```python
from build123d import *

# Parameters (mm, degrees)
SKETCH1_R           = 9.525
BOSS_EXTRUDE1_DEPTH = 76.2
SKETCH3_R           = 8.509
CUT_EXTRUDE1_DEPTH  = 1.524
SKETCH4_R           = 8.001
CUT_EXTRUDE2_DEPTH  = 75.676
SKETCH5_R           = 12.4206
CUT_EXTRUDE3_DEPTH  = 254


with BuildPart() as part:
    # Sketch1 → Boss-Extrude1 (new body)
    with BuildSketch(Plane(origin=(0, 0, 0), x_dir=(0, 0, -1), z_dir=(1, 0, 0))):
        Circle(SKETCH1_R)
    extrude(amount=BOSS_EXTRUDE1_DEPTH)

    # Sketch3 → Cut-Extrude1 (cut)
    with BuildSketch(Plane.ZY):
        Circle(SKETCH3_R)
    extrude(amount=-CUT_EXTRUDE1_DEPTH, mode=Mode.SUBTRACT)

    # Sketch4 → Cut-Extrude2 (cut, through all)
    with BuildSketch(Plane.ZY.offset(-1.524)):
        Circle(SKETCH4_R)
    extrude(amount=-CUT_EXTRUDE2_DEPTH, mode=Mode.SUBTRACT)

    # Sketch5 → Cut-Extrude3 (cut)
    with BuildSketch(Plane.XY.offset(9.525)):
        with Locations((76.2, 0)):
            Circle(SKETCH5_R)
    extrude(amount=-CUT_EXTRUDE3_DEPTH, mode=Mode.SUBTRACT)


solid = part.part
```
The model under review builds one solid part; all positions refer to its coordinate system, in mm. A direction names the side the tool comes from. Coordinates: 2 decimals unless noted, no trailing zeros. Write each loop counter-clockwise with the first axis right and the second up, starting at its lowest first coordinate (ties: lowest second). Pieces come first, ordered by that corner, then holes. Notation, with made-up numbers: (22.25, 47) -> (47.25, 47) arc R19 cw to (47.25, 81) -> close; hole circle Ø5 at (82.5, 20.5). An arc over 180 degrees is marked (long way). One line per item, written item: value. Start each with the question number.
Q1. Add section A-A, the plane y = 0. Give the boundary of the cut face in (x, z) (3 decimals), then the cut area to 3 significant figures.
Q2. Clearance check with flat-ended pins moving along their axes: P1, Ø3, axis at y = 2, z = -5, coming from the +X side; P2, Ø5, axis at x = 52.5, y = 6, coming from the +Z side; P3, Ø10, axis at y = 4, z = -4, coming from the +X side; P4, Ø4, axis at x = 48, y = 6.5, coming from the -Z side (3 decimals). State where each tip first meets the part, or that it passes through.
Q3. Add section C-C, the plane x = 63. Give the boundary of the cut face in (y, z) (3 decimals).
Q4. Add section B-B, the plane z = 0. Give the boundary of the cut face in (x, y) (3 decimals).
Q5. For faces 4 (the face through (33.66, -7.81, -1.73)), 5 (the face through (0.751, 8.437, -1.108)), list the 3-axis set-ups (+Z, -Z, +X, -X, +Y, -Y) from which the entire face can be reached by the end or side of a thin tool; tool diameter is ignored.
Q6. To check wall thickness, follow probe 1 along Y at (x, z) = (47, 0) (3 decimals); probe 2 along Y at (x, z) = (0.95, 0) (3 decimals). State the ranges of each line that lie inside material, in increasing order.
Q7. The part is to be moulded in two halves that separate along Y. For faces 1 (the face through (64.003, -2.348, 7.808)), 2 (the face through (33.64, -3.65, -8.8)), 3 (the face through (0, 8, 4)), say which applies: +Y half, -Y half, draft (parallel to the pull), parting line (faces both ways), or undercut.
Response:
1. outline: (0, -9.525) -> (63.779, -9.525) -> (63.779, -8.001) -> (1.524, -8.001) -> (1.524, -8.509) -> (0, -8.509) -> close; (0, 8.509) -> (1.524, 8.509) -> (1.524, 8.001) -> (63.779, 8.001) -> (63.779, 9.525) -> (0, 9.525) -> close
1. area: 193 mm²
2. P1: through
2. P2: z = 8.86
2. P3: x = 67.58
2. P4: z = -8.395
3. outline: circle Ø19.05 at (0, 0); hole circle Ø16.002 at (0, 0)
4. outline: (0, -9.525) -> (68.228, -9.525) arc R12.421 cw to (66.7, -8.001) -> (1.524, -8.001) -> (1.524, -8.509) -> (0, -8.509) -> close; (0, 8.509) -> (1.524, 8.509) -> (1.524, 8.001) -> (66.7, 8.001) arc R12.421 cw to (68.228, 9.525) -> (0, 9.525) -> close
5. face 4: +X, -X
5. face 5: -X
6. probe 1: -9.525 to -8.001, 8.001 to 9.525
6. probe 2: -9.525 to -8.509, 8.509 to 9.525
7. face 1: undercut
7. face 2: parting line
7. face 3: draft
